from build123d import *

# Parameters (mm, degrees)
SKETCH1_R           = 60
SKETCH1_R_2         = 50
BOSS_EXTRUDE2_DEPTH = 30
BOSS_EXTRUDE3_START = 10
SKETCH2_R           = 60
BOSS_EXTRUDE3_DEPTH = 10
SKETCH3_R           = 4.5
BOSS_EXTRUDE4_DEPTH = 10


with BuildPart() as part:
    # Sketch1 → Boss-Extrude2 (new body)
    with BuildSketch(Plane.XY):
        Circle(SKETCH1_R)
        Circle(SKETCH1_R_2, mode=Mode.SUBTRACT)
    extrude(amount=BOSS_EXTRUDE2_DEPTH)

    # Sketch2 → Boss-Extrude3 (add)
    with BuildSketch(Plane(origin=(0, 0, 0), x_dir=(-1, 0, 0), z_dir=(0, 0, -1)).offset(BOSS_EXTRUDE3_START)):
        Circle(SKETCH2_R)
    extrude(amount=-BOSS_EXTRUDE3_DEPTH)

    # Sketch3 → Boss-Extrude4 (add)
    with BuildSketch(Plane.XY):
        with Locations(Location((10.534503936, 0, 0), (0, 0, 180))):
            Circle(SKETCH3_R)
    extrude(amount=BOSS_EXTRUDE4_DEPTH)


solid = part.part
Read the model definition and answer for the solid it produces. Units are mm, in the model's axes. A direction names the side the tool comes from. Coordinates: 2 decimals unless noted, no trailing zeros. Loops run counter-clockwise (first coordinate to the right, second up) from the corner with the lowest first, then second, coordinate; pieces in that order, holes last.
Q1. The part is cut by section C-C on y = 0. Write down the section's boundary in (x, z).
Q2. The part is cut by section B-B on x = 0. Write down the section's boundary in (y, z), and give its area (3 significant figures).
Q3. The part is cut by section D-D on z = 21. Write down the section's boundary in (x, y).
Q4. The part is cut by section A-A on z = 6.5. Write down the section's boundary in (x, y), and give its area (3 significant figures).
Q5. Each of these flat-tipped pins is pushed along its axis until it touches: pin 1 Ø7 at (x, y) = (11.5, -0.5) entering from +Z; pin 2 Ø1 at (x, z) = (9.5, 3) entering from -Y; pin 3 Ø12 at (y, z) = (-10, 20.5) entering from +X. Where does it stop, or does it pass through?
Q6. Consider probe 1 along Y at (x, z) = (0, 14.25); probe 2 along Z at (x, y) = (32, 19.5); probe 3 along Y at (x, z) = (42, 22). Determine where each line is inside the solid, lowest interval first.
Q7. Which of the six approach directions +Z, -Z, +X, -X, +Y, -Y give full straight-line access (tool end or side, diameter ignored) to faces 1 (the face through (15.03, -0.2, 4.93)), 2 (the face through (-23, 45, 30))?
Results below:
1. outline: (-60, -10) - (60, -10) - (60, 30) - (50, 30) - (50, 0) - (15.03, 0) - (15.03, 10) - (6.03, 10) - (6.03, 0) - (-50, 0) - (-50, 30) - (-60, 30) - close
2. outline: (-60, -10) - (60, -10) - (60, 30) - (50, 30) - (50, 0) - (-50, 0) - (-50, 30) - (-60, 30) - close
2. area: 1,800 mm2
3. outline: circle Ø120 at (0, 0); hole circle Ø100 at (0, 0)
4. outline: circle Ø120 at (0, 0); circle Ø9 at (10.53, 0); hole circle Ø100 at (0, 0)
4. area: 3,520 mm2
5. pin 1: stops at z = 10
5. pin 2: stops at y = -59.32
5. pin 3: stops at x = 59.87
6. probe 1: y = -60 to -50, 50 to 60
6. probe 2: z = -10 to 0
6. probe 3: y = -42.85 to -27.13, 27.13 to 42.85
7. face 1: +Z
7. face 2: +Z, +X, -X, +Y, -Y
